Check sheet for the modelled part. Datum: model origin and axes. Units: mm. Face numbers are marked on the shaded views. A direction names the side the tool comes from. Coordinates: 2 decimals unless noted, no trailing zeros. Loops run counter-clockwise (first coordinate to the right, second up) from the corner with the lowest first, then second, coordinate; pieces in that order, holes last.
```python
from build123d import *

# Parameters (mm, degrees)
SKETCH1_W           = 100
SKETCH1_H           = 100
BOSS_EXTRUDE1_DEPTH = 100
CUT_EXTRUDE1_DEPTH  = 50
CIRPATTERN1_COUNT   = 4
SKETCH3_R           = 12.5
CUT_EXTRUDE2_DEPTH  = 50


with BuildPart() as part:
    # Sketch1 → Boss-Extrude1 (new body)
    with BuildSketch(Plane(origin=(0, 0, 0), x_dir=(1, 0, 0), z_dir=(0, 1, 0))):
        Rectangle(SKETCH1_W, SKETCH1_H)
    extrude(amount=BOSS_EXTRUDE1_DEPTH)

    # Sketch2 → Cut-Extrude1 (cut)
    with BuildSketch(Plane.XY.offset(50)):
        with BuildLine():
            Line((0, 14.113800065), (-26.260063577, 59.59756439))
            ThreePointArc((-26.260063577, 59.59756439), (-13.130031788, 72.727596179), (0, 59.59756439))
            ThreePointArc((0, 59.59756439), (13.130031788, 72.727596179), (26.260063577, 59.59756439))
            Line((26.260063577, 59.59756439), (0, 14.113800065))
        make_face()
    cut_extrude1 = extrude(amount=-CUT_EXTRUDE1_DEPTH, mode=Mode.SUBTRACT)

    # CirPattern1: Cut-Extrude1 ×4 about axis
    cirpattern1_axis = Axis((0, 0, 0), (0, 1, 0))
    for i in range(1, CIRPATTERN1_COUNT):
        add(cut_extrude1.rotate(cirpattern1_axis, i * 360 / CIRPATTERN1_COUNT), mode=Mode.SUBTRACT)

    # Sketch3 → Cut-Extrude2 (cut)
    with BuildSketch(Plane(origin=(0, 100, 0), x_dir=(1, 0, 0), z_dir=(0, 1, 0))):
        with Locations(Location((0, 0, 0), (0, 0, 270))):
            Circle(SKETCH3_R)
    extrude(amount=-CUT_EXTRUDE2_DEPTH, mode=Mode.SUBTRACT)


solid = part.part
```
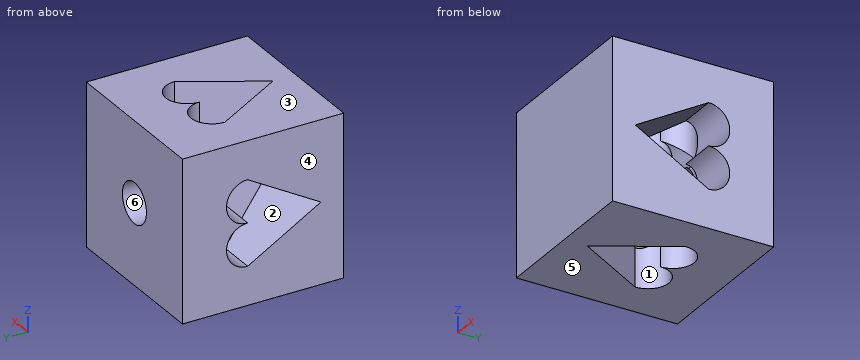
1) Section check B-B on z = 42. Enter the section's corners in (x, y).
Answer sheet:
outline: (-50, 0) - (50, 0) - (50, 100) - (-50, 100) - close; hole (-26.26, 59.6) - (0, 14.11) - (26.26, 59.6) arc R13.13 ccw to (0, 59.6) arc R13.13 ccw to start
2) Scan lines: line 1 (Z direction, x = 0, y = 88); line 2 (Z direction, x = 45, y = 66). Record each from-to range of solid material in increasing order.
Answer sheet:
line 1: z = -50 to -12.5, 12.5 to 50
line 2: z = -50 to -24.59, -1.67 to 1.67, 24.59 to 50
3) Depth check by flat-ended pin: pin 1 (1.5 mm diameter, centred on x = 0.5, z = 28, fed in from -Y). Enter the tip coordinate at first touch or a pass-through.
Answer sheet:
pin 1: stops at y = 0
4) Set-up check for the marked faces 1, 2 and 3: record each of +Z, -Z, +X, -X, +Y, -Y from which the full face is reachable in a straight line by a thin tool's end or side.
Answer sheet:
face 1: +Z, -Z
face 2: +X, -X
face 3: +Z, +X, -X, +Y, -Y
5) Mould release check, pull along Z, two halves, no side actions. Record for the marked faces 4, 5 and 6: +Z half, -Z half, draft (parallel to the pull), parting line (faces both ways), or undercut.
Answer sheet:
face 4: draft
face 5: -Z half
face 6: undercut
6) Section check A-A on x = -29. Enter the section's corners in (y, z), plus the area to 3 significant figures.
Answer sheet:
outline: (0, -50) - (100, -50) - (100, 50) - (0, 50) - close; hole (14.11, 0) - (59.6, -26.26) arc R13.13 ccw to (59.6, 0) arc R13.13 ccw to (59.6, 26.26) - close
area: 8,260 mm2
7) Section check C-C on y = 27.5. Enter the section's corners in (x, z), plus the area to 3 significant figures.
Answer sheet:
outline: (-50, -50) - (-7.73, -50) - (-7.73, -7.73) - (-50, -7.73) - close; (-50, 7.73) - (-7.73, 7.73) - (-7.73, 50) - (-50, 50) - close; (7.73, -50) - (50, -50) - (50, -7.73) - (7.73, -7.73) - close; (7.73, 7.73) - (50, 7.73) - (50, 50) - (7.73, 50) - close
area: 7,150 mm2
8) Section check D-D on z = 7. Enter the section's corners in (x, y).
Answer sheet:
outline: (-50, 0) - (50, 0) - (50, 26.24) - (7, 26.24) - (0, 14.11) - (-7, 26.24) - (-50, 26.24) - close; (-50, 71.21) - (-19.26, 71.21) arc R13.13 cw to (-10.36, 72.43) - (-10.36, 100) - (-50, 100) - close; (10.36, 72.43) arc R13.13 cw to (19.26, 71.21) - (50, 71.21) - (50, 100) - (10.36, 100) - close
